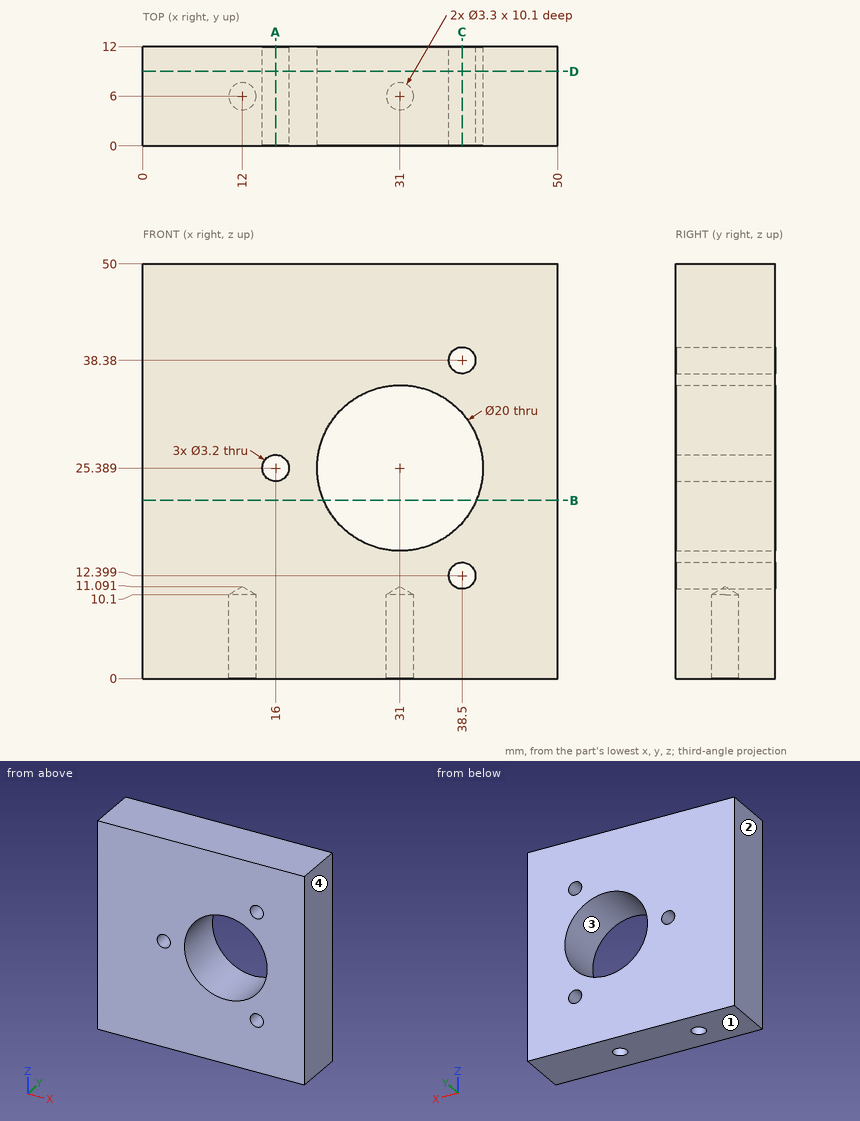
Design review of the part shown in the three views and the two pictorial views. Dimensions are in mm from the part's minimum x, y and z. Round coordinates to 2 decimals unless told otherwise and drop trailing zeros. Order: outer loops, then holes, each group sorted by start corner. A loop starts at its lowest first (then second) coordinate and runs counter-clockwise, first axis right, second up. Notation, with made-up numbers: M 2.5,54 L 47.5,54 A19 ccw 47.5,64 Z; hole C 12.5,-3.5 d7. An arc over 180 degrees is marked long. Put each result on its own line as item: value.
Q1. Consider section B-B (z = 21.5). State the section outline as (x, y) points.
Reported:
outline: M 0,0 L 21.79,0 L 21.79,12 L 0,12 Z; M 40.21,0 L 50,0 L 50,12 L 40.21,12 Z
Q2. Consider section C-C (x = 38.5). State the section outline as (y, z) points (1 decimal).
Reported:
outline: M 0,0 L 12,0 L 12,10.8 L 0,10.8 Z; M 0,14 L 12,14 L 12,18.8 L 0,18.8 Z; M 0,32 L 12,32 L 12,36.8 L 0,36.8 Z; M 0,40 L 12,40 L 12,50 L 0,50 Z
Q3. Consider section A-A (x = 16). State the section outline as (y, z) points.
Reported:
outline: M 0,0 L 12,0 L 12,23.79 L 0,23.79 Z; M 0,26.99 L 12,26.99 L 12,50 L 0,50 Z
Q4. Insertion check: pin 1 Ø12 at (x, z) = (12.5, 5.5) entering from -Y. The pin has a flat end and moves straight along its axis. Give the tip position at first contact, or say it passes through.
Reported:
pin 1: y = 0
Q5. Draft analysis for pull direction X (two halves, no side actions). For the marked faces 1, 2, 3 and 4, state which applies: released by +X, released by -X, zero draft, split by the parting line, or undercut.
Reported:
face 1: zero draft
face 2: released by -X
face 3: undercut
face 4: released by +X
Q6. Consider section D-D (y = 9). State the section outline as (x, z) points.
Reported:
outline: M 0,0 L 50,0 L 50,50 L 0,50 Z; hole C 16,25.39 d3.2; hole C 31,25.39 d20; hole C 38.5,12.4 d3.2; hole C 38.5,38.38 d3.2
Q7. To check wall thickness, follow line 1 (X direction, y = 6, z = 8); line 2 (Z direction, x = 38.5, y = 3) (1 decimal); line 3 (Z direction, x = 16, y = 2). State the ranges of each line that lie inside material, in increasing order.
Reported:
line 1: 0 to 10.35, 13.65 to 29.35, 32.65 to 50
line 2: 0 to 10.8, 14 to 18.8, 32 to 36.8, 40 to 50
line 3: 0 to 23.79, 26.99 to 50
